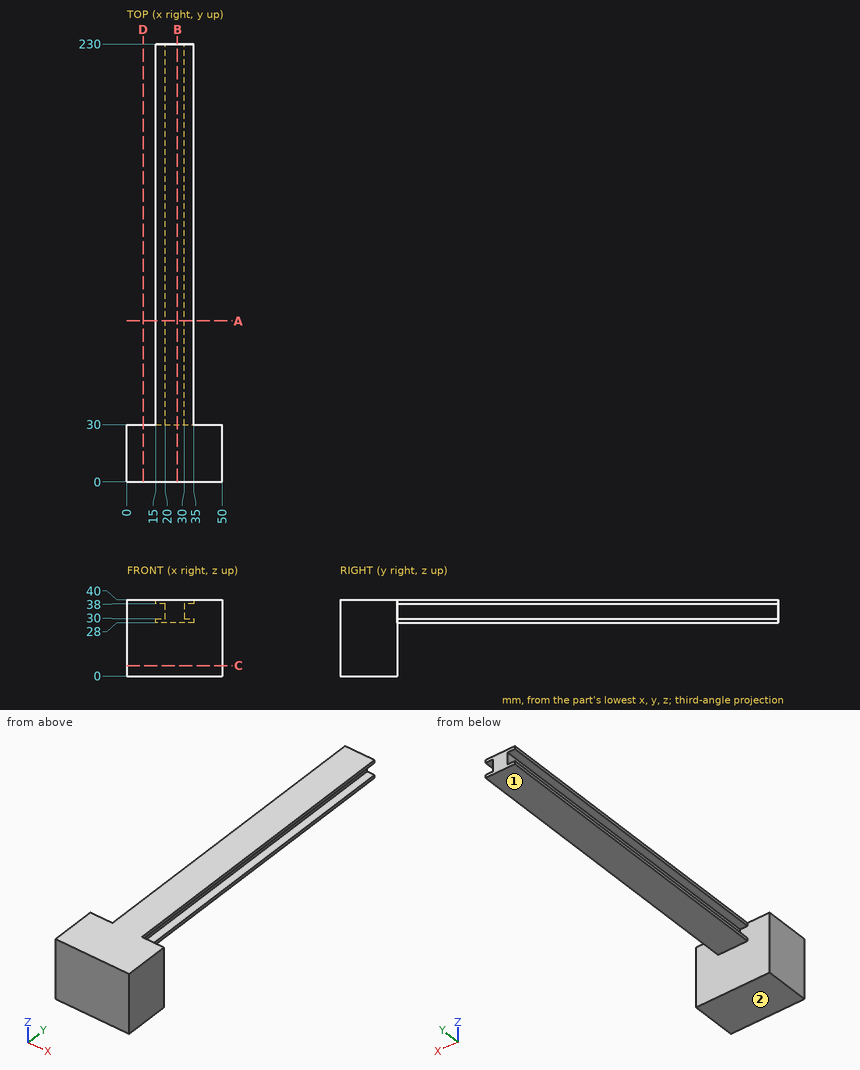
Geometry check sheet. Reference: drawing and pictorial views, mm from the part's lowest x, y, z. A direction names the side the tool comes from. Coordinates: 2 decimals unless noted, no trailing zeros. Order: outer loops, then holes, each group sorted by start corner. A loop starts at its lowest first (then second) coordinate and runs counter-clockwise, first axis right, second up.
Item 1: Tool access check on the marked faces 1 and 2. Record the directions out of +Z, -Z, +X, -X, +Y, -Y that give a thin tool (end or side, any length) a straight path to the whole face; none if there is none.
Item 2: Section check C-C (z = 5.5). Enter the section's corners in (x, y).
Item 3: Section check B-B (x = 26.5). Enter the section's corners in (y, z), plus the area to 3 significant figures.
Item 4: Depth check by flat-ended pin: pin 1 (5.5 mm diameter, centred on x = 16.5, y = 126.5, fed in from -Z); pin 2 (12 mm diameter, centred on y = 36.5, z = 26.5, fed in from -X); pin 3 (4 mm diameter, centred on y = 137, z = 32.5, fed in from +X). Enter the tip coordinate at first touch or a pass-through.
Item 5: Scan lines: line 1 along Z through (x, y) = (18.5, 65.5); line 2 along Y through (x, z) = (41, 24.5); line 3 along Z through (x, y) = (24.5, 181). Record each from-to range of solid material in increasing order.
Item 6: Section check D-D (x = 8.5). Enter the section's corners in (y, z), plus the area to 3 significant figures.
Item 7: Section check A-A (y = 84.5). Enter the section's corners in (x, z).
Check sheet entries:
1. face 1: -Z, +X, -X, +Y
1. face 2: -Z, +X, -X, +Y, -Y
2. outline: (0, 0) - (50, 0) - (50, 30) - (0, 30) - close
3. outline: (0, 0) - (30, 0) - (30, 28) - (230, 28) - (230, 40) - (0, 40) - close
3. area: 3,600 mm2
4. pin 1: stops at z = 28
4. pin 2: stops at x = 15
4. pin 3: stops at x = 30
5. line 1: z = 28 to 30, 38 to 40
5. line 2: y = 0 to 30
5. line 3: z = 28 to 40
6. outline: (0, 0) - (30, 0) - (30, 40) - (0, 40) - close
6. area: 1,200 mm2
7. outline: (15, 28) - (35, 28) - (35, 30) - (30, 30) - (30, 38) - (35, 38) - (35, 40) - (15, 40) - (15, 38) - (20, 38) - (20, 30) - (15, 30) - close
